Read the model definition and answer for the solid it produces. Units are mm, in the model's axes. Face numbers are marked on the shaded views. A direction names the side the tool comes from. Round coordinates to 2 decimals unless told otherwise and drop trailing zeros. Write each loop counter-clockwise with the first axis right and the second up, starting at its lowest first coordinate (ties: lowest second). Pieces come first, ordered by that corner, then holes.
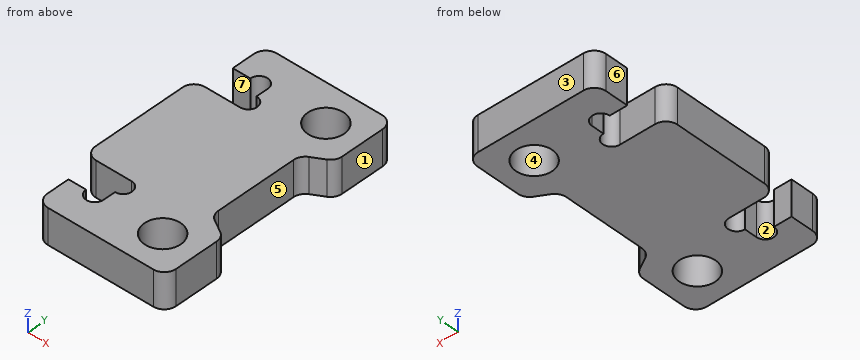
from build123d import *

# Parameters (mm, degrees)
SKETCH_1_R          = 1.55
EXTRUDE_1_DEPTH     = 1.5
SKETCH_2_W          = 3
SKETCH_2_H          = 2.95
SKETCH_2_W_2        = 4
SKETCH_2_H_2        = 10
EXTRUDE_2_DEPTH     = 3
SKETCH_3_R          = 0.75
CUT_EXTRUDE_1_DEPTH = 4
FILLET_1_R          = 1


with BuildPart() as part:
    # 草图1 → 凸台-拉伸1 (new body, symmetric)
    with BuildSketch(Plane.XY):
        Polygon((-5, 10.5), (-5, -10.5), (3, -10.5), (3, -5.190598923), (1, -4.035898385), (1, 4.035898385), (3, 5.190598923), (3, 10.5), align=None)
        with Locations((0, 7.5)):
            Circle(SKETCH_1_R, mode=Mode.SUBTRACT)
        with Locations((0, -7.5)):
            Circle(SKETCH_1_R, mode=Mode.SUBTRACT)
    extrude(amount=EXTRUDE_1_DEPTH, both=True)

    # 草图2 → 凸台-拉伸2 (add)
    with BuildSketch(Plane.XY.offset(1.5)):
        with Locations((-6.5, -9.025)):
            Rectangle(SKETCH_2_W, SKETCH_2_H)
        with Locations((-7, 0)):
            Rectangle(SKETCH_2_W_2, SKETCH_2_H_2)
        with Locations((-6.5, 9.025)):
            Rectangle(SKETCH_2_W, SKETCH_2_H)
    extrude(amount=-EXTRUDE_2_DEPTH)

    # 草图3 → 切除-拉伸1 (cut, through all)
    with BuildSketch(Plane.XY.offset(1.5)):
        with Locations((-5.75, 7.55)):
            Circle(SKETCH_3_R)
        with Locations((-5, 5.75)):
            Circle(SKETCH_3_R)
        with Locations((-5, -5.75)):
            Circle(SKETCH_3_R)
        with Locations((-5.75, -7.55)):
            Circle(SKETCH_3_R)
    extrude(amount=-CUT_EXTRUDE_1_DEPTH, mode=Mode.SUBTRACT)

    # 圆角1
    fillet_1_edges = [part.edges().sort_by_distance(p)[0] for p in [
        (3, 10.5, 0),
        (3, 5.190598923, 0),
        (1, 4.035898385, 0),
        (1, -4.035898385, 0),
        (3, -5.190598923, 0),
        (3, -10.5, 0),
        (-8, 10.5, 0),
        (-8, -10.5, 0),
        (-9, 5, 0),
        (-9, -5, 0),
    ]]
    fillet(fillet_1_edges, radius=FILLET_1_R)


solid = part.part
Q1. Flat-ended cylindrical pins translate along their axes: pin 1 Ø1 at (y, z) = (-8.5, 0.5) entering from -X; pin 2 Ø2.5 at (x, y) = (0, 7.5) entering from -Z; pin 3 Ø0.5 at (y, z) = (7, -0.5) entering from -X; pin 4 Ø0.8 at (x, z) = (-7.5, 0) entering from -Y (3 decimals). Find the tip coordinate at first contact, or state that the pin passes through.
Verdict:
pin 1: stops at x = -8
pin 2: passes through
pin 3: stops at x = -5
pin 4: stops at y = -10.495
Q2. Section A-A (x = 0) is taken. Determine the outline of the cut face in (y, z).
Verdict:
outline: (-10.5, -1.5) - (-9.05, -1.5) - (-9.05, 1.5) - (-10.5, 1.5) - close; (-5.95, -1.5) - (5.95, -1.5) - (5.95, 1.5) - (-5.95, 1.5) - close; (9.05, -1.5) - (10.5, -1.5) - (10.5, 1.5) - (9.05, 1.5) - close
Q3. Section B-B (z = 0.35) is taken. State how many separate pieces and enclosed holes the cut face has, then the cut area to 3 significant figures.
Verdict:
separate pieces: 1
enclosed holes: 2
area: 187 mm2
Q4. Section C-C (y = 8.75) is taken. Determine the outline of the cut face in (x, z).
Verdict:
outline: (-8, -1.5) - (-0.92, -1.5) - (-0.92, 1.5) - (-8, 1.5) - close; (0.92, -1.5) - (3, -1.5) - (3, 1.5) - (0.92, 1.5) - close
Q5. Determine the mould class of the marked faces 1, 2, 3 and 4 for opening direction Y: pulls with the +Y half, pulls with the -Y half, needs draft (parallel to the pull), parting line crosses it, or undercut.
Verdict:
face 1: needs draft
face 2: undercut
face 3: pulls with the +Y half
face 4: undercut
Q6. Section D-D (x = -5.75) is taken. Determine the outline of the cut face in (y, z).
Verdict:
outline: (-10.5, -1.5) - (-8.3, -1.5) - (-8.3, 1.5) - (-10.5, 1.5) - close; (-5, -1.5) - (5, -1.5) - (5, 1.5) - (-5, 1.5) - close; (8.3, -1.5) - (10.5, -1.5) - (10.5, 1.5) - (8.3, 1.5) - close
Q7. Straight lines are drawn through the part: probe 1 along Y at (x, z) = (0, -0.55); probe 2 along Y at (x, z) = (1.25, 0.3); probe 3 along Y at (x, z) = (-0.75, -0.9). For each, find the intervals that lie inside material, in ascending order.
Verdict:
probe 1: y = -10.5 to -9.05, -5.95 to 5.95, 9.05 to 10.5
probe 2: y = -10.5 to -8.42, -6.58 to -4.12, 4.12 to 6.58, 8.42 to 10.5
probe 3: y = -10.5 to -8.86, -6.14 to 6.14, 8.86 to 10.5
Q8. Which of the six approach directions +Z, -Z, +X, -X, +Y, -Y give full straight-line access (tool end or side, diameter ignored) to the marked faces 5, 6 and 7?
Verdict:
face 5: +Z, -Z, +X
face 6: +Z, -Z, -X, +Y
face 7: +Z, -Z, -X
